Model file for the job. Use its own axes, mm. Round coordinates to 2 decimals unless told otherwise and drop trailing zeros. Loops run counter-clockwise (first coordinate to the right, second up) from the corner with the lowest first, then second, coordinate; pieces in that order, holes last.
Autodesk Inventor part; units mm, degrees
ref_plane "YZ Plane" through (0, 0, 0) normal (1, 0, 0) x (0, 1, 0)
ref_plane "XZ Plane" through (0, 0, 0) normal (0, 1, 0) x (-1, 0, 0)
ref_plane "XY Plane" through (0, 0, 0) normal (0, 0, 1) x (1, 0, 0)
sketch "Sketch1" plane through (0, 0, 0) normal (0, 1, 0) x (-1, 0, 0)
  line L0 (0, 0) -> (100, 0)
  line L1 (100, 0) -> (100, -110)
  line L2 (100, -110) -> (0, -110)
  line L3 (0, -110) -> (0, 0)
  dimension "d0" = 100
  dimension "d1" = 110
extrude "Extrusion1" add sketch "Sketch1" along normal blind 5
sketch "Sketch2" plane through (0, 5, 0) normal (0, 1, 0) x (1, 0, 0)
  circle A0 centre (-7, 13.8333) radius 4.5
  line L0 (0, 0) -> (0, 110)
  line L1 (-100, 0) -> (0, 0)
  circle A1 centre (-7, 55.3333) radius 4.5
  circle A2 centre (-7, 96.8333) radius 4.5
  line L2 (-34, 0) -> (-34, 110)
  circle A3 centre (-61, 13.8333) radius 4.5
  circle A4 centre (-61, 55.3333) radius 4.5
  circle A5 centre (-61, 96.8333) radius 4.5
  circle A6 centre (-82.6974, 13.8333) radius 3
  dimension "d4" = 9
  dimension "d5" = 7
  dimension "d6" = 110
  dimension "d7" = 13.8333
  dimension "d10" = 41.5
  dimension "d19" = 27
  dimension "d20" = 6
extrude "Extrusion2" cut sketch "Sketch2" against normal blind 10
sketch "Sketch3" plane through (0, 5, 0) normal (0, 1, 0) x (1, 0, 0)
  line L0 (-100, 110) -> (0, 110)
  line L1 (-100, 110) -> (0, 110)
  line L2 (0, 110) -> (0, 160)
  line L3 (0, 160) -> (-100, 160)
  line L4 (-100, 160) -> (-100, 110)
  point P0 (0, 0)
  dimension "d21" = 50
extrude "Extrusion3" add sketch "Sketch3" against normal blind 5
equation "\"d7\" = -0.5 * d4 + 0.166667 * d6"
equation "\"d10\" = -1.5 * d4 + 0.5 * d6"
properties part number "HeaderWheelSupport"
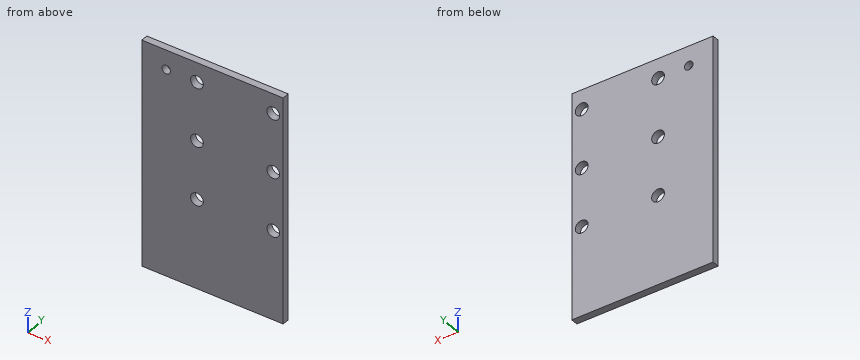
Q1. Slice it at B-B on y = 1.3. Give the cut face in (x, z).
Q2. Slice it at A-A on x = -7. Give the cut face in (y, z).
Q3. Probe line 1 (Z direction, x = -7, y = 2.45); line 2 (X direction, y = 2.95, z = -12); line 3 (Z direction, x = -85, y = 4.75). List the from-to ranges inside material, lowest first.
Reply:
1. outline: (-100, -160) - (0, -160) - (0, 0) - (-100, 0) - close; hole circle Ø6 at (-82.7, -13.83); hole circle Ø9 at (-61, -96.83); hole circle Ø9 at (-61, -55.33); hole circle Ø9 at (-61, -13.83); hole circle Ø9 at (-7, -96.83); hole circle Ø9 at (-7, -55.33); hole circle Ø9 at (-7, -13.83)
2. outline: (0, -160) - (5, -160) - (5, -101.33) - (0, -101.33) - close; (0, -92.33) - (5, -92.33) - (5, -59.83) - (0, -59.83) - close; (0, -50.83) - (5, -50.83) - (5, -18.33) - (0, -18.33) - close; (0, -9.33) - (5, -9.33) - (5, 0) - (0, 0) - close
3. line 1: z = -160 to -101.33, -92.33 to -59.83, -50.83 to -18.33, -9.33 to 0
3. line 2: x = -100 to -85.07, -80.32 to -65.11, -56.89 to -11.11, -2.89 to 0
3. line 3: z = -160 to -15.76, -11.91 to 0
